Could you check a few things on this drawing? It's one solid part, dimensions in mm from its lowest x, y, z. A direction names the side the tool comes from. Give positions to 0.01 mm unless a question says otherwise; leave off trailing zeros. Write each loop counter-clockwise with the first axis right and the second up, starting at its lowest first coordinate (ties: lowest second). Pieces come first, ordered by that corner, then holes. Notation, with made-up numbers: (-8.75, 35) -> (10.25, 35) arc R22 ccw to (10.25, 44) -> close; hole circle Ø11 at (37, 6.25). An arc over 180 degrees is marked (long way). Answer as CSV lines item,"result". Start each with the question number.
1. If we section it at D-D on z = 103: Write out the boundary of the cut face in (x, y) (1 decimal), plus the area to 3 significant figures.
2. I'm going to push flat-ended pins straight in: P1, Ø8.5, axis at y = 42.5, z = 5, coming from the +X side; P2, Ø6, axis at y = 27, z = 110, coming from the -X side; P3, Ø6, axis at x = 109, y = 15.5, coming from the -Z side. Where does each tip first touch, or does it pass through?
3. I need wall thicknesses on line 1 (X direction, y = 61, z = 116.5) (1 decimal); line 2 (Y direction, x = 52, z = 115.5); line 3 (Z direction, x = 81, y = 45) (1 decimal). Which ranges of each line are inside material? Lowest first, please. Write a range as [from, to].
4. On a 3-axis mill with a long thin cutter (end or side, diameter ignored), from which of +Z, -Z, +X, -X, +Y, -Y can I reach the whole of each face in a straight line? I mean the marked faces 1 and 2. Say none if no direction works.
5. If we mould it in two halves opening along Z, with no side actions, what happens to the marked faces 3, 4, 5 and 6? For each: pulls with the +Z half, pulls with the -Z half, needs draft (parallel to the pull), parting line crosses it, or undercut.
6. If we section it at B-B on z = 65: Write out the boundary of the cut face in (x, y).
7. If we section it at C-C on x = 107.5: Write out the boundary of the cut face in (y, z) (1 decimal).
8. If we section it at A-A on y = 36: Write out the boundary of the cut face in (x, z) (1 decimal).
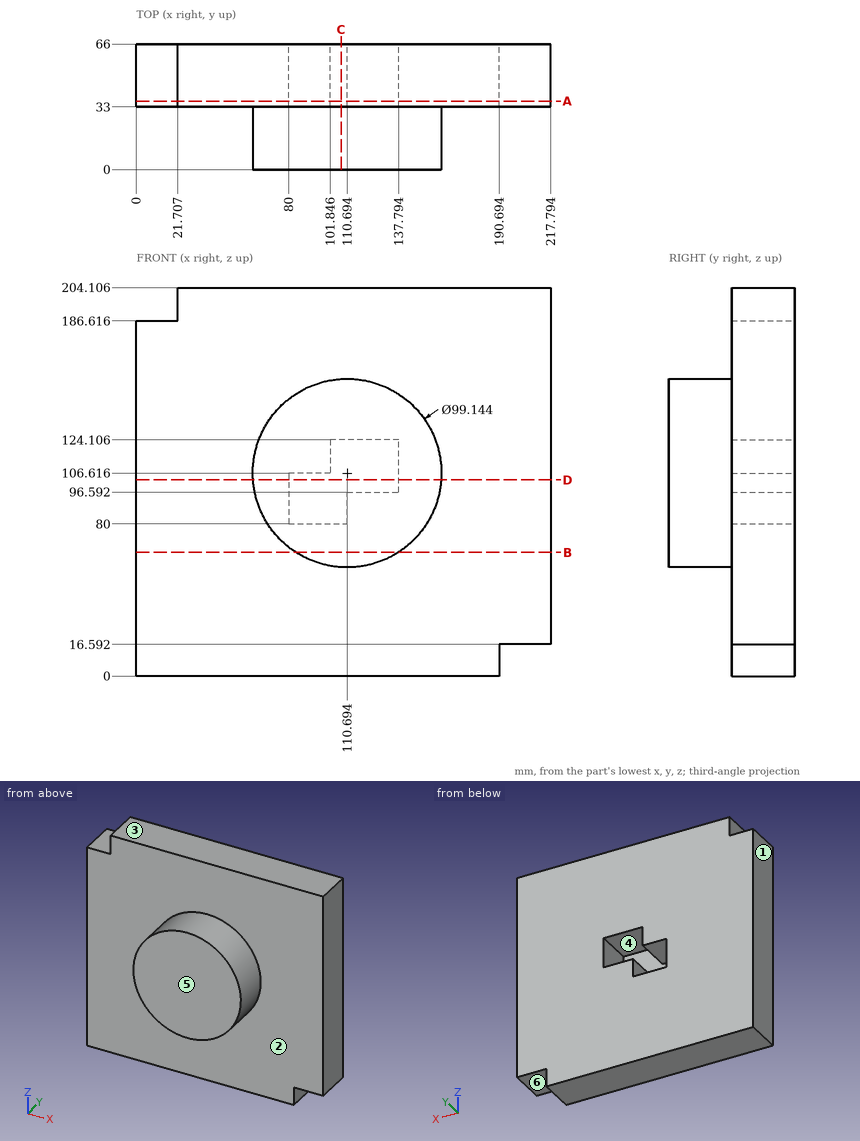
Computed values:
1,outline,"(0, 33) -> (61.3, 33) -> (61.3, 0) -> (160.1, 0) -> (160.1, 33) -> (217.8, 33) -> (217.8, 66) -> (137.8, 66) -> (137.8, 33) -> (80, 33) -> (80, 66) -> (0, 66) -> close"
1,area,"8,540 mm2"
2,P1,"stops at x = 190.69"
2,P2,"stops at x = 61.12"
2,P3,"stops at z = 57.04"
3,line 1,"x = [0, 101.8], [137.8, 217.8]"
3,line 2,"y = [33, 66]"
3,line 3,"z = [0, 80], [106.6, 204.1]"
4,face 1,"+Z, -Z, -X, +Y, -Y"
4,face 2,"-Y"
5,face 3,"pulls with the +Z half"
5,face 4,"undercut"
5,face 5,"needs draft"
5,face 6,"pulls with the -Z half"
6,outline,"(0, 33) -> (83.76, 33) -> (83.76, 0) -> (137.63, 0) -> (137.63, 33) -> (217.79, 33) -> (217.79, 66) -> (0, 66) -> close"
7,outline,"(0, 57.1) -> (33, 57.1) -> (33, 0) -> (66, 0) -> (66, 80) -> (33, 80) -> (33, 124.1) -> (66, 124.1) -> (66, 204.1) -> (33, 204.1) -> (33, 156.1) -> (0, 156.1) -> close"
8,outline,"(0, 0) -> (190.7, 0) -> (190.7, 16.6) -> (217.8, 16.6) -> (217.8, 204.1) -> (21.7, 204.1) -> (21.7, 186.6) -> (0, 186.6) -> close; hole (80, 80) -> (110.7, 80) -> (110.7, 96.6) -> (137.8, 96.6) -> (137.8, 124.1) -> (101.8, 124.1) -> (101.8, 106.6) -> (80, 106.6) -> close"
